CAD build for the part. Positions are in the model's coordinates, mm. A direction names the side the tool comes from. Give positions to 0.01 mm unless a question says otherwise; leave off trailing zeros. Write each loop counter-clockwise with the first axis right and the second up, starting at its lowest first coordinate (ties: lowest second). Pieces come first, ordered by that corner, then holes. Notation, with made-up numbers: (-8.5, 26.5) - (-2.5, 26.5) arc R23 cw to (-2.5, 65.5) - close; hole circle Ø4 at (56, -8.5). An arc over 180 degrees is marked (long way). Answer as a JSON object with one key per item and string values.
from build123d import *

# Parameters (mm, degrees)
F0_R     = 19.05
F1_DEPTH = 196.85
F2_R     = 6.35
F3_DEPTH = 25.4
F4_R     = 6.35
F5_DEPTH = 25.4


with BuildPart() as f1:
    # F0 (on Front) → F1 (new body, symmetric)
    with BuildSketch(Plane.XZ):
        Circle(F0_R)
    extrude(amount=F1_DEPTH, both=True)

    # F2 (on face) → F3 (join)
    with BuildSketch(Plane(origin=(0, 196.85, 0), x_dir=(-1, 0, 0), z_dir=(0, 1, 0))):
        Circle(F2_R)
    extrude(amount=F3_DEPTH)

    # F4 (on face) → F5 (join)
    with BuildSketch(Plane.XZ.offset(196.85)):
        Circle(F4_R)
    extrude(amount=F5_DEPTH)


solid = f1.part
(1) Saw through at C-C, the plane y = -70.5. Give the cut face in (x, z), and give its area (3 significant figures).
Answer key:
{"outline": "circle Ø38.1 at (0, 0)", "area": "1,140 mm²"}
(2) Flat gauge pins, fed straight in: P1, Ø10, axis at x = -3, y = -134, coming from the +Z side; P2, Ø5, axis at x = 13.5, y = -15.5, coming from the -Z side; P3, Ø8, axis at x = -10.5, z = -10.5, coming from the +Y side; P4, Ø4, axis at x = -5.5, z = 4.5, coming from the -Y side. Where does each tip first touch, or does it go through?
Answer key:
{"P1": "stops at z = 19.05", "P2": "stops at z = -15.55", "P3": "stops at y = 196.85", "P4": "stops at y = -222.25"}
(3) 3-axis set-ups, long thin cutter, end or side, ignore diameter. For faces 3 (the face through (1.38, 209.37, -6.2)), 4 (the face through (-15.12, -2.76, -11.59)): which of +Z, -Z, +X, -X, +Y, -Y reach the whole face in a straight line?
Answer key:
{"face 3": "+Y", "face 4": "+Y, -Y"}
(4) Probe L1, parallel to Y at x = 4.5, z = -8; L2, parallel to Z at x = 0, y = 161; L3, parallel to X at y = 49.5, z = 0.5. List the from-to ranges inside material, lowest first. Write a range as [from, to].
Answer key:
{"L1": "y = [-196.85, 196.85]", "L2": "z = [-19.05, 19.05]", "L3": "x = [-19.04, 19.04]"}
(5) Saw through at A-A, the plane x = 0. Give the cut face in (y, z), and give its area (3 significant figures).
Answer key:
{"outline": "(-222.25, -6.35) - (-196.85, -6.35) - (-196.85, -19.05) - (196.85, -19.05) - (196.85, -6.35) - (222.25, -6.35) - (222.25, 6.35) - (196.85, 6.35) - (196.85, 19.05) - (-196.85, 19.05) - (-196.85, 6.35) - (-222.25, 6.35) - close", "area": "15,600 mm²"}
(6) Pull direction Z, two halves, no side cores. Call faces 1 (the face through (-1.38, -209.37, -6.2)), 2 (the face through (-5, -196.85, 5)): pulls with the +Z half, pulls with the -Z half, needs draft (parallel to the pull), parting line crosses it, or undercut.
Answer key:
{"face 1": "parting line crosses it", "face 2": "needs draft"}
(7) Saw through at B-B, the plane z = 0. Give the cut face in (x, y).
Answer key:
{"outline": "(-19.05, -196.85) - (-6.35, -196.85) - (-6.35, -222.25) - (6.35, -222.25) - (6.35, -196.85) - (19.05, -196.85) - (19.05, 196.85) - (6.35, 196.85) - (6.35, 222.25) - (-6.35, 222.25) - (-6.35, 196.85) - (-19.05, 196.85) - close"}
